Here's how the part is built. I have some questions about the finished solid (model axes, mm). Face numbers are marked on the shaded views. A direction names the side the tool comes from. Coordinates: 2 decimals unless noted, no trailing zeros. Loops run counter-clockwise (first coordinate to the right, second up) from the corner with the lowest first, then second, coordinate; pieces in that order, holes last. Notation, with made-up numbers: (82.25, 67) -> (136.25, 67) arc R10 ccw to (136.25, 71) -> close; hole circle Ø8 at (27.5, 19). An arc over 180 degrees is marked (long way). Answer as a JSON object with one key per item and string values. Group by question number.
Q1. I want a section at A-A on x = 5. Write out the boundary of the cut face in (y, z).
Q2. I want a section at C-C on x = 3.75. Write out the boundary of the cut face in (y, z), then the cut area to 3 significant figures.
Q3. Thinking about a two-plate mould opening in X: for the marked faces 1, 2 and 3, which applies, released by +X, released by -X, zero draft, split by the parting line, or undercut?
Q4. I want a section at B-B on y = 2.75. Write out the boundary of the cut face in (x, z), then the cut area to 3 significant figures.
Q5. I need wall thicknesses on line 1 (Y direction, x = 7.54, z = 8.25); line 2 (X direction, y = 1.75, z = 1); line 3 (X direction, y = 3.75, z = 9.25). Which ranges of each line are inside material? Lowest first, please.
Q6. I want a section at D-D on z = 7.75. Write out the boundary of the cut face in (x, y), then the cut area to 3 significant figures.
Q7. On a 3-axis mill with a long thin cutter (end or side, diameter ignored), from which of +Z, -Z, +X, -X, +Y, -Y can I reach the whole of each face in a straight line? I mean the marked faces 4, 5, 6 and 7. Say none if no direction works.
Q8. I'm going to push flat-ended pins straight in: pin 1 (2.5 mm diameter, centred on x = 6.5, z = 11, fed in from +Y); pin 2 (1.8 mm diameter, centred on y = 2.5, z = 10.5, fed in from -X); pin 3 (2 mm diameter, centred on x = 4, y = 3, fed in from -Z). Where does each tip first touch, or does it pass through?
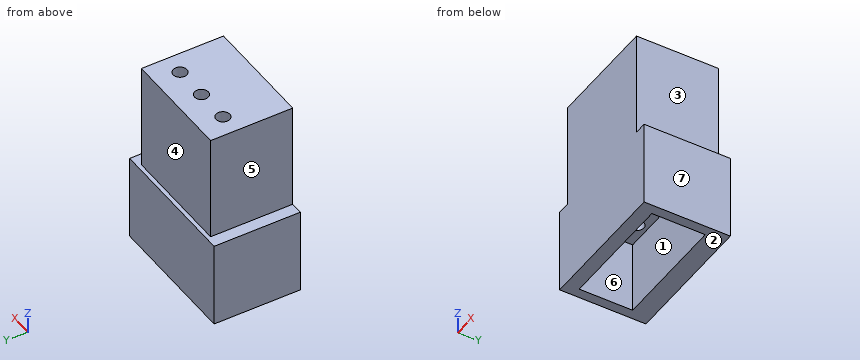
```python
from build123d import *

# Parameters (mm, degrees)
SKETCH_1_W               = 10
SKETCH_1_H               = 6.3
SKETCH_1_W_2             = 8.6
SKETCH_1_H_2             = 3.9
EXTRUDE_1_DEPTH          = 6.3
SKETCH_2_W               = 8.2
SKETCH_2_H               = 6
EXTRUDE_2_DEPTH          = 7.8
SKETCH_3_W               = 10
SKETCH_3_H               = 6.3
EXTRUDE_3_DEPTH          = 1
CUT_EXTRUDE_1_DEPTH      = 19.398369493
CUT_EXTRUDE_1_DEPTH_BACK = 19.398369493
SKETCH_4_R               = 0.5


with BuildPart() as part:
    # 草图1 → 凸台-拉伸1 (new body)
    with BuildSketch(Plane.XY):
        with Locations((5, 3.15)):
            Rectangle(SKETCH_1_W, SKETCH_1_H)
        with Locations((5, 2.95)):
            Rectangle(SKETCH_1_W_2, SKETCH_1_H_2, mode=Mode.SUBTRACT)
    extrude(amount=EXTRUDE_1_DEPTH)

    # 草图2 → 凸台-拉伸2 (add)
    with BuildSketch(Plane.XY.offset(6.3)):
        with Locations((5, 3)):
            Rectangle(SKETCH_2_W, SKETCH_2_H)
    extrude(amount=EXTRUDE_2_DEPTH)

    # 草图3 → 凸台-拉伸3 (add)
    with BuildSketch(Plane(origin=(0, 0, 6.3), x_dir=(-1, 0, 0), z_dir=(0, 0, -1))):
        with Locations((-5, 3.15)):
            Rectangle(SKETCH_3_W, SKETCH_3_H)
    extrude(amount=EXTRUDE_3_DEPTH)

    # 草图4 → 切除-拉伸1 (cut, two sides: drawn at the far end of the back side and taken through both)
    with BuildSketch(Plane.XY.offset(14.1).offset(-CUT_EXTRUDE_1_DEPTH_BACK)):
        with Locations((2.46, 4.138210579)):
            Circle(SKETCH_4_R)
        with Locations((5, 4.138210579)):
            Circle(SKETCH_4_R)
        with Locations((7.54, 4.138210579)):
            Circle(SKETCH_4_R)
    extrude(amount=CUT_EXTRUDE_1_DEPTH + CUT_EXTRUDE_1_DEPTH_BACK, mode=Mode.SUBTRACT)


solid = part.part
```
Result set:
{
 "1": {"outline": "(0, 0) -> (1, 0) -> (1, 5.3) -> (3.64, 5.3) -> (3.64, 14.1) -> (0, 14.1) -> close; (4.64, 5.3) -> (4.9, 5.3) -> (4.9, 0) -> (6.3, 0) -> (6.3, 6.3) -> (6, 6.3) -> (6, 14.1) -> (4.64, 14.1) -> close"},
 "2": {"outline": "(0, 0) -> (1, 0) -> (1, 5.3) -> (4.9, 5.3) -> (4.9, 0) -> (6.3, 0) -> (6.3, 6.3) -> (6, 6.3) -> (6, 14.1) -> (0, 14.1) -> close", "area": "65.8 mm²"},
 "3": {"face 1": "undercut", "face 2": "zero draft", "face 3": "released by +X"},
 "4": {"outline": "(0, 0) -> (0.7, 0) -> (0.7, 5.3) -> (9.3, 5.3) -> (9.3, 0) -> (10, 0) -> (10, 6.3) -> (9.1, 6.3) -> (9.1, 14.1) -> (0.9, 14.1) -> (0.9, 6.3) -> (0, 6.3) -> close", "area": "81.4 mm²"},
 "5": {"line 1": "y = 0 to 3.64, 4.64 to 6", "line 2": "x = 0 to 0.7, 9.3 to 10", "line 3": "x = 0.9 to 2.14, 2.78 to 4.68, 5.32 to 7.22, 7.86 to 9.1"},
 "6": {"outline": "(0.9, 0) -> (9.1, 0) -> (9.1, 6) -> (0.9, 6) -> close; hole circle Ø1 at (2.46, 4.14); hole circle Ø1 at (5, 4.14); hole circle Ø1 at (7.54, 4.14)", "area": "46.8 mm²"},
 "7": {"face 4": "+Z, +X, -X, +Y", "face 5": "+Z, -X, +Y, -Y", "face 6": "-Z", "face 7": "+Z, -Z, +X, +Y, -Y"},
 "8": {"pin 1": "stops at y = 6", "pin 2": "stops at x = 0.9", "pin 3": "stops at z = 5.3"}
}
